Can you work these out from the model? Positions are in its coordinate system, mm. A direction names the side the tool comes from. Coordinates: 2 decimals unless noted, no trailing zeros. Write each loop counter-clockwise with the first axis right and the second up, starting at its lowest first coordinate (ties: lowest second). Pieces come first, ordered by that corner, then holes.
Autodesk Inventor part; units mm, degrees
ref_plane "YZ Plane" through (0, 0, 0) normal (1, 0, 0) x (0, 1, 0)
ref_plane "XZ Plane" through (0, 0, 0) normal (0, 1, 0) x (-1, 0, 0)
ref_plane "XY Plane" through (0, 0, 0) normal (0, 0, 1) x (1, 0, 0)
sketch "Esboço1" plane through (0, 0, 0) normal (0, 0, 1) x (1, 0, 0)
  line L0 (-59, 10.75) -> (43.5, 10.75)
  line L1 (43.5, 10.75) -> (43.5, -22)
  line L2 (43.5, -22) -> (-59, -22)
  line L3 (-59, -22) -> (-59, 10.75)
  point P0 (0, 0)
  dimension "d34" = 43.5
  dimension "d35" = 22
  dimension "d49" = 10.75
  dimension "d59" = 59
extrude "Extrusão1" add sketch "Esboço1" along normal blind 3
sketch "Esboço2" plane through (0, 0, 3) normal (0, 0, 1) x (1, 0, 0)
  line L0 (-59, -22) -> (43.5, -22)
  line L1 (43.5, -22) -> (42.5, -22)
  line L2 (43.5, 10.75) -> (26.875, 10.75)
  line L3 (26.875, 10.75) -> (26.875, 6.75)
  line L4 (26.875, 6.75) -> (43.5, 6.75)
  line L5 (43.5, 6.75) -> (43.5, 10.75)
  line L6 (14.875, 10.75) -> (-1.75, 10.75)
  line L7 (-1.75, 10.75) -> (-1.75, 6.75)
  line L8 (-1.75, 6.75) -> (14.875, 6.75)
  line L9 (14.875, 6.75) -> (14.875, 10.75)
  line L10 (-13.75, 10.75) -> (-30.375, 10.75)
  line L11 (-30.375, 10.75) -> (-30.375, 6.75)
  line L12 (-30.375, 6.75) -> (-13.75, 6.75)
  line L13 (-13.75, 6.75) -> (-13.75, 10.75)
  line L14 (-42.375, 10.75) -> (-59, 10.75)
  line L15 (-59, 10.75) -> (-59, 6.75)
  line L16 (-59, 6.75) -> (-42.375, 6.75)
  line L17 (-42.375, 6.75) -> (-42.375, 10.75)
  line L18 (43.5, -22) -> (32.6, -22)
  line L19 (32.6, -22) -> (32.6, -18)
  line L20 (32.6, -18) -> (43.5, -18)
  line L21 (43.5, -18) -> (43.5, -22)
  line L22 (9.7, -22) -> (9.7, -18)
  line L23 (20.6, -22) -> (19.6, -22)
  line L24 (20.6, -22) -> (9.7, -22)
  line L25 (20.6, -18) -> (20.6, -22)
  line L26 (9.7, -18) -> (20.6, -18)
  line L27 (-13.2, -22) -> (-13.2, -18)
  line L28 (-2.3, -22) -> (-3.3, -22)
  line L29 (-2.3, -22) -> (-13.2, -22)
  line L30 (-2.3, -18) -> (-2.3, -22)
  line L31 (-13.2, -18) -> (-2.3, -18)
  line L32 (-36.1, -22) -> (-36.1, -18)
  line L33 (-25.2, -22) -> (-26.2, -22)
  line L34 (-25.2, -22) -> (-36.1, -22)
  line L35 (-25.2, -18) -> (-25.2, -22)
  line L36 (-36.1, -18) -> (-25.2, -18)
  line L37 (-59, -22) -> (-59, -18)
  line L38 (-48.1, -22) -> (-49.1, -22)
  line L39 (-48.1, -22) -> (-59, -22)
  line L40 (-48.1, -18) -> (-48.1, -22)
  line L41 (-59, -18) -> (-48.1, -18)
  line L42 (-59, 10.75) -> (-59, -22)
  line L43 (-59, -22) -> (-59, -22)
  line L44 (-59, -22) -> (-59, -18)
  line L45 (-59, -18) -> (-59, -18)
  line L46 (-59, -18) -> (-59, -22)
  line L47 (-59, 6.75) -> (-59, 6.75)
  line L48 (-59, 6.75) -> (-59, 10.75)
  line L49 (-59, 10.75) -> (-59, 10.75)
  line L50 (-59, 10.75) -> (-59, 6.75)
  line L51 (-59, -18) -> (-59, -9.625) construction
  line L52 (-59, -9.625) -> (-55, -9.625) construction
  line L53 (-55, 2.375) -> (-59, 2.375) construction
  line L54 (-59, 2.375) -> (-59, -9.625) construction
  line L55 (-13.75, 10.75) -> (-13.75, -22) construction
  line L56 (43.5, -22) -> (43.5, 10.75)
  line L57 (43.5, -9.625) -> (39.5, -9.625) construction
  line L58 (39.5, -1.625) -> (43.5, -1.625) construction
  line L59 (43.5, -1.625) -> (43.5, -9.625)
  line L60 (39.5, -9.625) -> (43.5, -9.625)
  line L61 (43.5, -9.625) -> (43.5, -18)
  line L62 (43.5, -18) -> (39.5, -18)
  line L63 (39.5, -18) -> (39.5, -9.625)
  line L64 (39.5, -1.625) -> (43.5, -1.625)
  line L65 (43.5, -1.625) -> (43.5, 6.75)
  line L66 (43.5, 6.75) -> (39.5, 6.75)
  line L67 (39.5, 6.75) -> (39.5, -1.625)
  line L68 (-55, -9.625) -> (-59, -9.625)
  line L69 (-59, -9.625) -> (-59, -18)
  line L70 (-59, -18) -> (-55, -18)
  line L71 (-55, -18) -> (-55, -9.625)
  line L72 (-55, 2.375) -> (-59, 2.375)
  line L73 (-59, 2.375) -> (-59, 6.75)
  line L74 (-59, 6.75) -> (-55, 6.75)
  line L75 (-55, 6.75) -> (-55, 2.375)
  point P0 (-48.1, -22)
  point P1 (-36.1, -22)
  point P2 (-25.2, -22)
  point P3 (-13.2, -22)
  point P4 (-2.3, -22)
  point P5 (9.7, -22)
  point P6 (32.6, -22)
  point P7 (-57.4, -18)
  point P8 (-57, 14.75)
  point P9 (-59, 10.75)
  point P10 (-55, 6.75)
  point P11 (-59, 6.75)
  point P12 (39.5, 6.75)
  point P13 (43.5, -1.625)
  dimension "d40" = 4
  dimension "d41" = 16.625
  dimension "d44" = 28.625
  dimension "d50" = 10.9
  dimension "d51" = 4
  dimension "d54" = 22.9
  dimension "d60" = 8.375
extrude "Extrusão2" cut sketch "Esboço2" against normal through all
properties part number "Acrilico-Parachoque"
1. Which directions (+Z, -Z, +X, -X, +Y, -Y) give clear straight access to the entire face, cutting with the end or side of a thin tool? Please do faces 1 (the face through (-30.375, 9, 2)), 2 (the face through (-52, -18, 2)), 3 (the face through (41, -1.625, 2)).
2. If I drill on L1, parallel to X at y = 9, z = 2.4 (3 decimals); L2, parallel to X at y = -19.5, z = 2.05; L3, parallel to Y at x = 6.5, z = 2.2, over which ranges is the centre line in solid material (lowest first)?
3. I'm going to push flat-ended pins straight in: P1, Ø1.5, axis at y = 8.5, z = 2, coming from the +X side (3 decimals); P2, Ø1, axis at x = 4, z = 0.5, coming from the +Y side; P3, Ø1.5, axis at x = -52.5, z = 1, coming from the -Y side. Where does each tip first touch, or does it pass through?
4. If we section it at B-B, the plane x = 3.5: List the corners of the cut face in (y, z) for me, plus the area to 4 significant figures.
5. If we section it at A-A, the plane y = -13: List the corners of the cut face in (x, z) for me.
6. We'd pull the mould along X, two halves only. Please class faces 4 (the face through (36, -18, 2)), 5 (the face through (43.5, -6, 1)), 6 (the face through (-1.75, 9, 2)): released by +X, released by -X, zero draft, split by the parting line, or undercut.
Answers:
1. face 1: +Z, -Z, +Y
1. face 2: +Z, -Z, -X, -Y
1. face 3: +Z, -Z, +X, +Y
2. L1: x = -42.375 to -30.375, -13.75 to -1.75, 14.875 to 26.875
2. L2: x = -48.1 to -36.1, -25.2 to -13.2, -2.3 to 9.7, 20.6 to 32.6
2. L3: y = -22 to 6.75
3. P1: stops at x = 26.875
3. P2: stops at y = 6.75
3. P3: stops at y = -18
4. outline: (-22, 0) - (6.75, 0) - (6.75, 3) - (-22, 3) - close
4. area: 86.25 mm2
5. outline: (-55, 0) - (39.5, 0) - (39.5, 3) - (-55, 3) - close
6. face 4: zero draft
6. face 5: released by +X
6. face 6: undercut
